Source: three-view drawing plus pictorial views. Frame: mm from the lowest corner of the part. Give positions to 0.01 mm unless a question says otherwise; leave off trailing zeros. Order: outer loops, then holes, each group sorted by start corner. A loop starts at its lowest first (then second) coordinate and runs counter-clockwise, first axis right, second up. Notation, with made-up numbers: (-23, -27) -> (-6, -27) arc R27 ccw to (-6, -11) -> close; hole circle Ø3 at (41.25, -6.5). An arc over 180 degrees is marked (long way). Answer in a Markdown table with one row per item. Add a question column.
Q1. Cut plane C-C on y = 1.45. Return the cut outline in (x, z).
Q2. Cut plane D-D on x = 25. Return the cut outline in (y, z), and give its area (3 significant figures).
Q3. Line query: line 1 along X through (y, z) = (1.05, 49) (1 decimal); line 2 along Z through (x, y) = (22, 1.6); line 3 along X through (y, z) = (1.65, 36.5) (1 decimal). Output: solid intervals per line, ascending. Write a range as from..to.
Q4. Contact query for flat-ended pins moving along their axis: P1, Ø1.5, axis at y = 1, z = 54.5, coming from the -X side; P2, Ø2.5, axis at x = 46, z = 15, coming from the +Y side; P3, Ø1.5, axis at y = 2.5, z = 48.5, coming from the -X side (1 decimal); P4, Ø1.5, axis at x = 39.5, y = 1.5, coming from the -Z side. Output: stop coordinate, or through.
Q5. Cut plane A-A on x = 14. Return the cut outline in (y, z), and give its area (3 significant figures).
Q6. Cut plane B-B on z = 52. Return the cut outline in (x, y).
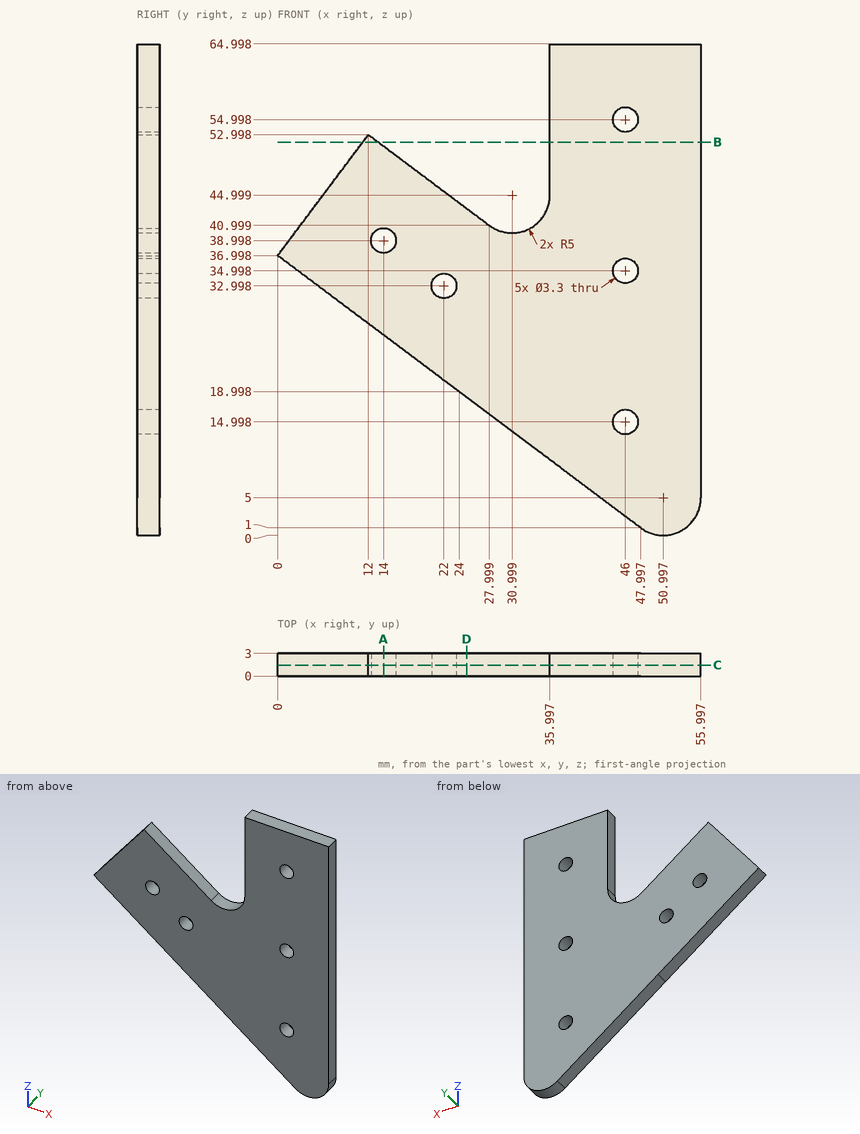
Completed:
| question | item | result |
|---|---|---|
| 1 | outline | (0, 37) -> (48, 1) arc R5 ccw to (56, 5) -> (56, 65) -> (36, 65) -> (36, 45) arc R5 cw to (28, 41) -> (12, 53) -> close; hole circle Ø3.3 at (14, 39); hole circle Ø3.3 at (22, 33); hole circle Ø3.3 at (46, 15); hole circle Ø3.3 at (46, 35); hole circle Ø3.3 at (46, 55) |
| 2 | outline | (0, 18.25) -> (3, 18.25) -> (3, 43.25) -> (0, 43.25) -> close |
| 2 | area | 75.0 mm² |
| 3 | line 1 | x = 9..17.3, 36..56 |
| 3 | line 2 | z = 20.5..31.35, 34.65..45.5 |
| 3 | line 3 | x = 0.7..45.3, 46.7..56 |
| 4 | P1 | stops at x = 36 |
| 4 | P2 | passes through |
| 4 | P3 | stops at x = 8.1 |
| 4 | P4 | stops at z = 6.81 |
| 5 | outline | (0, 26.5) -> (3, 26.5) -> (3, 37.35) -> (0, 37.35) -> close; (0, 40.65) -> (3, 40.65) -> (3, 51.5) -> (0, 51.5) -> close |
| 5 | area | 65.1 mm² |
| 6 | outline | (11.25, 0) -> (13.33, 0) -> (13.33, 3) -> (11.25, 3) -> close; (36, 0) -> (56, 0) -> (56, 3) -> (36, 3) -> close |
